Verification items for the finished model (mm, model axes). Face numbers are marked on the shaded views. A direction names the side the tool comes from. Round coordinates to 2 decimals unless told otherwise and drop trailing zeros. Order: outer loops, then holes, each group sorted by start corner. A loop starts at its lowest first (then second) coordinate and runs counter-clockwise, first axis right, second up. Notation, with made-up numbers: M 32.5,54.5 L 74.5,54.5 A16 ccw 74.5,69.5 Z; hole C 44.5,51.5 d8. An arc over 180 degrees is marked long. One line per item, written item: value. Start each with the question number.
from build123d import *

# Parameters (mm, degrees)
BOSS_EXTRUDE1_DEPTH = 2
BOSS_EXTRUDE2_START = 0.5
BOSS_EXTRUDE2_DEPTH = 4


with BuildPart() as part:
    # Sketch1 → Boss-Extrude1 (new body)
    with BuildSketch(Plane(origin=(0, 0, 0), x_dir=(1, 0, 0), z_dir=(0, 1, 0))):
        with BuildLine():
            Line((-31.018542474, -5.25), (31.018542474, -5.25))
            ThreePointArc((31.018542474, -5.25), (31.712537746, -4.962537746), (32, -4.268542474))
            Line((32, -4.268542474), (32, 4.268542474))
            ThreePointArc((32, 4.268542474), (31.712537746, 4.962537746), (31.018542474, 5.25))
            Line((31.018542474, 5.25), (-31.018542474, 5.25))
            ThreePointArc((-31.018542474, 5.25), (-31.712537746, 4.962537746), (-32, 4.268542474))
            Line((-32, 4.268542474), (-32, -4.268542474))
            ThreePointArc((-32, -4.268542474), (-31.712537746, -4.962537746), (-31.018542474, -5.25))
        make_face()
        with BuildLine():
            Line((-26.215, 3.50000032), (-26.215, -3.50000032))
            ThreePointArc((-26.215, -3.50000032), (-26.068553391, -3.853553711), (-25.715, -4.00000032))
            Line((-25.715, -4.00000032), (25.715, -4.00000032))
            ThreePointArc((25.715, -4.00000032), (26.068553391, -3.853553711), (26.215, -3.50000032))
            Line((26.215, -3.50000032), (26.215, 3.50000032))
            ThreePointArc((26.215, 3.50000032), (26.068553391, 3.853553711), (25.715, 4.00000032))
            Line((25.715, 4.00000032), (-25.715, 4.00000032))
            ThreePointArc((-25.715, 4.00000032), (-26.068553391, 3.853553711), (-26.215, 3.50000032))
        make_face(mode=Mode.SUBTRACT)
    extrude(amount=BOSS_EXTRUDE1_DEPTH)

    # Sketch2 → Boss-Extrude2 (add)
    with BuildSketch(Plane(origin=(0, 0, 0), x_dir=(1, 0, 0), z_dir=(0, 1, 0)).offset(BOSS_EXTRUDE2_START)):
        with BuildLine():
            Line((-31.018542474, -7.25), (31.018542474, -7.25))
            ThreePointArc((31.018542474, -7.25), (33.126751308, -6.376751308), (34, -4.268542474))
            Line((34, -4.268542474), (34, 4.268542474))
            ThreePointArc((34, 4.268542474), (33.126751308, 6.376751308), (31.018542474, 7.25))
            Line((31.018542474, 7.25), (-31.018542474, 7.25))
            ThreePointArc((-31.018542474, 7.25), (-33.126751308, 6.376751308), (-34, 4.268542474))
            Line((-34, 4.268542474), (-34, -4.268542474))
            ThreePointArc((-34, -4.268542474), (-33.126751308, -6.376751308), (-31.018542474, -7.25))
        make_face()
        with BuildLine():
            Line((-31.018542474, -5.25), (31.018542474, -5.25))
            ThreePointArc((31.018542474, -5.25), (31.712537746, -4.962537746), (32, -4.268542474))
            Line((32, -4.268542474), (32, 4.268542474))
            ThreePointArc((32, 4.268542474), (31.712537746, 4.962537746), (31.018542474, 5.25))
            Line((31.018542474, 5.25), (-31.018542474, 5.25))
            ThreePointArc((-31.018542474, 5.25), (-31.712537746, 4.962537746), (-32, 4.268542474))
            Line((-32, 4.268542474), (-32, -4.268542474))
            ThreePointArc((-32, -4.268542474), (-31.712537746, -4.962537746), (-31.018542474, -5.25))
        make_face(mode=Mode.SUBTRACT)
    extrude(amount=-BOSS_EXTRUDE2_DEPTH)


solid = part.part
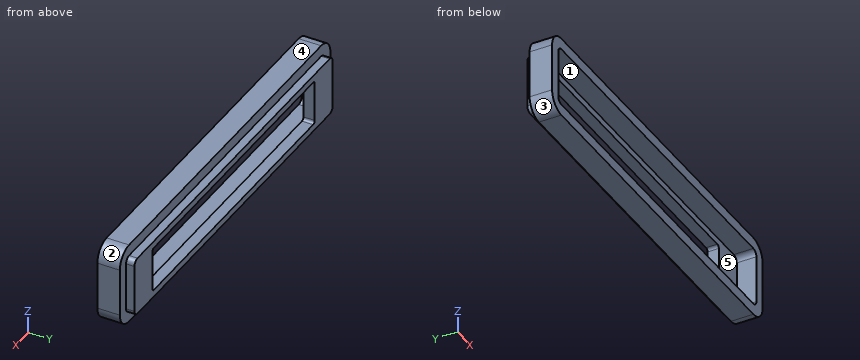
1. Tool access check on the marked faces 4 and 5. Record the directions out of +Z, -Z, +X, -X, +Y, -Y that give a thin tool (end or side, any length) a straight path to the whole face; none if there is none.
2. Scan lines: line 1 along Z through (x, y) = (-4, -0.8); line 2 along Z through (x, y) = (16, 0.3); line 3 along X through (y, z) = (-2.25, 1.75). Record each from-to range of solid material in increasing order.
3. Draft check along X on the marked faces 1, 2 and 3. Enter one of: released by +X, released by -X, zero draft, split by the parting line, or undercut.
4. Section check C-C (x = -2). Record the cut outline in (y, z), and give its area (3 significant figures).
5. Section check B-B (z = -1.75). Record the cut outline in (x, y) (3 decimals), and give its area (3 significant figures).
6. Depth check by flat-ended pin: pin 1 (1 mm diameter, centred on x = -15.5, z = -2, fed in from +Y); pin 2 (1.6 mm diameter, centred on y = 1.5, z = -1.5, fed in from +X); pin 3 (5.5 mm diameter, centred on x = 5.5, z = 2, fed in from -Y); pin 4 (1.6 mm diameter, centred on y = 1.5, z = 1, fed in from -X). Enter the tip coordinate at first touch or a pass-through.
7. Section check A-A (y = -1). Record the cut outline in (x, z).
Geometry check:
1. face 4: +Z, +X, -X, +Y, -Y
1. face 5: -Y
2. line 1: z = -7.25 to -5.25, 5.25 to 7.25
2. line 2: z = -7.25 to -4, 4 to 7.25
2. line 3: x = -34 to -32, 32 to 34
3. face 1: undercut
3. face 2: released by +X
3. face 3: released by -X
4. outline: M -3.5,-7.25 L 0.5,-7.25 L 0.5,-5.25 L 2,-5.25 L 2,-4 L 0,-4 L 0,-5.25 L -3.5,-5.25 Z; M -3.5,5.25 L 0,5.25 L 0,4 L 2,4 L 2,5.25 L 0.5,5.25 L 0.5,7.25 L -3.5,7.25 Z
4. area: 21.0 mm²
5. outline: M -34,-3.5 L -32,-3.5 L -32,0 L -26.215,0 L -26.215,2 L -32,2 L -32,0.5 L -34,0.5 Z; M 26.215,0 L 32,0 L 32,-3.5 L 34,-3.5 L 34,0.5 L 32,0.5 L 32,2 L 26.215,2 Z
5. area: 39.1 mm²
6. pin 1: passes through
6. pin 2: stops at x = 32
6. pin 3: stops at y = 0
6. pin 4: stops at x = -32
7. outline: M -34,-4.27 A2.98 ccw -31.02,-7.25 L 31.02,-7.25 A2.98 ccw 34,-4.27 L 34,4.27 A2.98 ccw 31.02,7.25 L -31.02,7.25 A2.98 ccw -34,4.27 Z; hole M -32,-4.27 A0.98 ccw -31.02,-5.25 L 31.02,-5.25 A0.98 ccw 32,-4.27 L 32,4.27 A0.98 ccw 31.02,5.25 L -31.02,5.25 A0.98 ccw -32,4.27 Z
